Part model, mm, in its own coordinate system. Round coordinates to 2 decimals unless told otherwise and drop trailing zeros. Loops run counter-clockwise (first coordinate to the right, second up) from the corner with the lowest first, then second, coordinate; pieces in that order, holes last. Notation, with made-up numbers: (76.5, -21) -> (135.5, -21) arc R9 ccw to (135.5, -15) -> close; hole circle Ø10 at (30.25, 8.25). An arc over 180 degrees is marked (long way). Use a Markdown table: item, result. Add a question column.
Item 1: Cut at D-D, the plane z = -62. List the corners of the cut face in (x, y) (3 decimals).
Item 2: Probe line 1 (Z direction, x = 6.25, y = 1); line 2 (X direction, y = 0.5, z = -18.5); line 3 (X direction, y = 2.25, z = 49). List the from-to ranges inside material, lowest first. Write a range as [from, to].
Item 3: Flat gauge pins, fed straight in: pin 1 (5 mm diameter, centred on y = 3, z = 26.5, fed in from +X); pin 2 (2 mm diameter, centred on y = 4.5, z = 3.5, fed in from -X). Where does each tip first touch, or does it go through?
Item 4: Cut at B-B, the plane z = 3. List the corners of the cut face in (x, y) (3 decimals).
Item 5: Cut at C-C, the plane x = 7.75. List the corners of the cut face in (y, z), plus the area to 3 significant figures.
Item 6: Cut at A-A, the plane y = 4.75. List the corners of the cut face in (x, z).
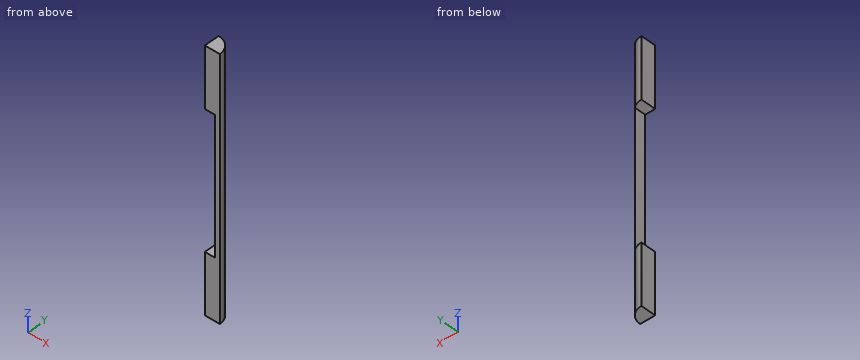
Autodesk Inventor part; units mm, degrees
ref_plane "YZ Plane" through (0, 0, 0) normal (1, 0, 0) x (0, 1, 0)
ref_plane "XZ Plane" through (0, 0, 0) normal (0, 1, 0) x (-1, 0, 0)
ref_plane "XY Plane" through (0, 0, 0) normal (0, 0, 1) x (1, 0, 0)
sketch "Sketch1" plane through (0, 0, 0) normal (0, 0, 1) x (1, 0, 0)
  arc A0 (9.525, 0) -> (0, 9.525) centre (0, 0) ccw
  line L0 (0, 9.525) -> (0, 0)
  line L1 (0, 0) -> (9.525, 0)
  dimension "d0" = 19.05
extrude "Extrusion1" add sketch "Sketch1" along normal mid plane 161.925
sketch "Sketch2" plane through (0, 0, 80.9625) normal (0, -1, 0) x (1, 0, 0)
  line L0 (0, -38.1) -> (6.35, -38.1)
  line L1 (6.35, -38.1) -> (6.35, -123.825)
  line L2 (6.35, -123.825) -> (0, -123.825)
  line L3 (0, -123.825) -> (0, -38.1)
  line L4 (9.525, -161.925) -> (0, -161.925)
  line L5 (0, -161.925) -> (0, 0)
  point P0 (0, -80.9625)
  dimension "d3" = 85.725
  dimension "d4" = 38.1
  dimension "d5" = 6.35
extrude "Extrusion2" cut sketch "Sketch2" against normal through all
equation "\"d0\" = cornerRoundType"
equation "\"d1\" = lengthOfPart"
equation "\"d3\" = notchCutout"
equation "\"d4\" = bottomLength"
equation "\"cornerRoundType\" = 19.05"
equation "\"notchCutout\" = 85.725"
equation "\"bottomLength\" = 38.1"
equation "\"lengthOfPart\" = 2 * bottomLength + notchCutout"
properties part number "topOfStairs"
A:
| question | item | result |
|---|---|---|
| 1 | outline | (0, 0) -> (9.525, 0) arc R9.525 ccw to (0, 9.525) -> close |
| 2 | line 1 | z = [-80.96, -42.86], [42.86, 80.96] |
| 2 | line 2 | x = [6.35, 9.51] |
| 2 | line 3 | x = [0, 9.26] |
| 3 | pin 1 | stops at x = 9.51 |
| 3 | pin 2 | stops at x = 6.35 |
| 4 | outline | (6.35, 0) -> (9.525, 0) arc R9.525 ccw to (6.35, 7.1) -> close |
| 5 | outline | (0, -80.96) -> (5.54, -80.96) -> (5.54, 80.96) -> (0, 80.96) -> close |
| 5 | area | 897 mm^2 |
| 6 | outline | (0, -80.96) -> (8.26, -80.96) -> (8.26, 80.96) -> (0, 80.96) -> (0, 42.86) -> (6.35, 42.86) -> (6.35, -42.86) -> (0, -42.86) -> close |
